Answer from the drawing. Dimensions are ordinates in mm from the lowest x, y and z of the part. Round coordinates to 2 decimals unless told otherwise and drop trailing zeros. Order: outer loops, then holes, each group sorted by start corner. A loop starts at its lowest first (then second) coordinate and runs counter-clockwise, first axis right, second up. Notation, with made-up numbers: (-3, 70) - (44, 70) arc R19 ccw to (44, 100) - close; hole circle Ø5 at (54.25, 61). An arc over 180 degrees is marked (long way). One line per question, with ' | ' between items. Start each with the question number.
1) The part is cut by section C-C, the plane x = 17. Give the vertices of the cut face in (y, z) (1 decimal).
2) Flat-ended cylindrical pins translate along their axes: pin 1 (5 mm diameter, centred on x = 22.5, z = 5, fed in from -Y); pin 2 (1.2 mm diameter, centred on x = 30, y = 1.5, fed in from -Z). Find the tip coordinate at first contact, or state that the pin passes through.
3) The mould has two halves that part along X. Classify the marked faces 1, 2 and 3: pulls with the +X half, pulls with the -X half, needs draft (parallel to the pull), parting line crosses it, or undercut.
4) The part is cut by section A-A, the plane x = 25. Give the vertices of the cut face in (y, z).
5) Straight lines are drawn through the part: line 1 (Z direction, x = 20, y = 1.75); line 2 (X direction, y = 1.1, z = 15.25) (1 decimal); line 3 (X direction, y = 2.3, z = 19.25) (1 decimal). For each, find the intervals that lie inside material, in ascending order. Write a range as from..to.
6) The part is cut by section B-B, the plane z = 14.75. Give the vertices of the cut face in (x, y) (1 decimal), plus the area to 3 significant figures.
7) The part is cut by section D-D, the plane y = 0.8. Count the separate pieces of the cut face and the enclosed holes in it.
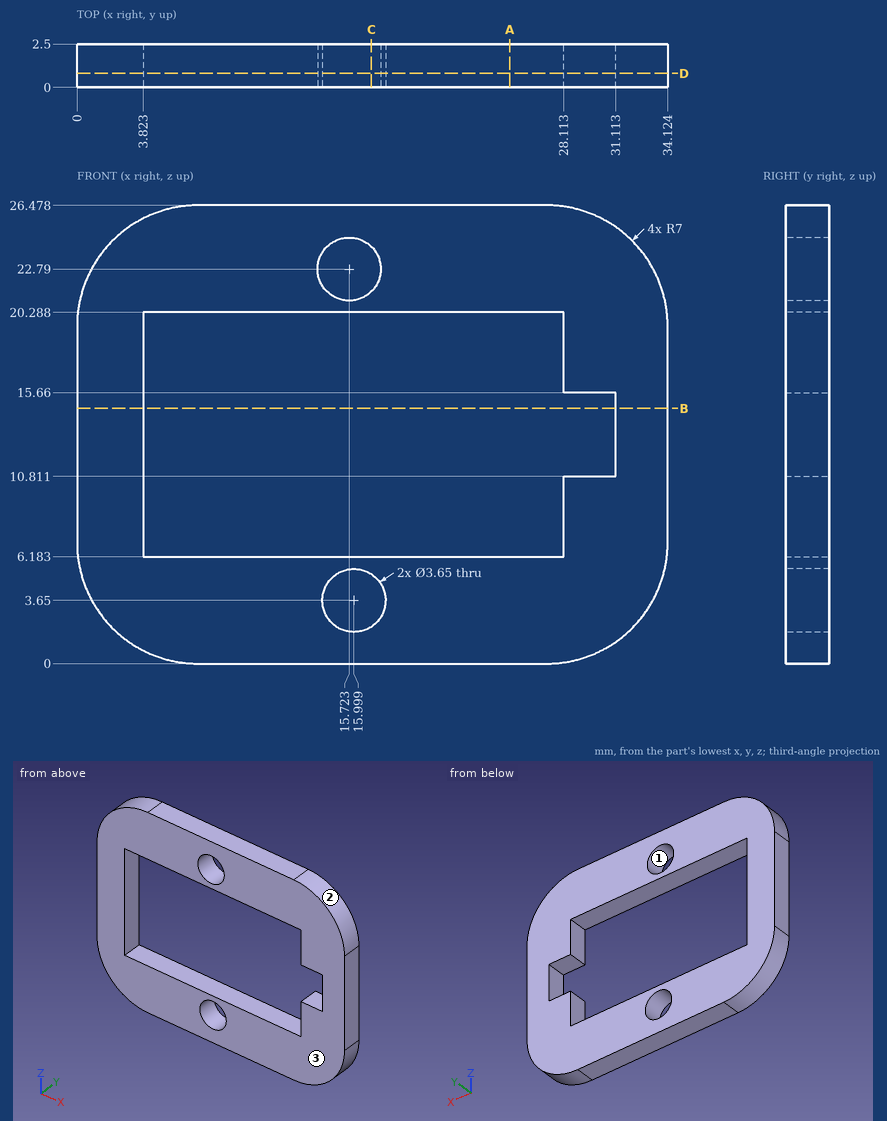
Values:
1) outline: (0, 0) - (2.5, 0) - (2.5, 2.1) - (0, 2.1) - close; (0, 5.2) - (2.5, 5.2) - (2.5, 6.2) - (0, 6.2) - close; (0, 20.3) - (2.5, 20.3) - (2.5, 21.5) - (0, 21.5) - close; (0, 24.1) - (2.5, 24.1) - (2.5, 26.5) - (0, 26.5) - close
2) pin 1: stops at y = 0 | pin 2: stops at z = 0.38
3) face 1: undercut | face 2: pulls with the +X half | face 3: needs draft
4) outline: (0, 0) - (2.5, 0) - (2.5, 6.18) - (0, 6.18) - close; (0, 20.29) - (2.5, 20.29) - (2.5, 26.48) - (0, 26.48) - close
5) line 1: z = 0..6.18, 20.29..26.48 | line 2: x = 0..3.8, 31.1..34.1 | line 3: x = 0..3.8, 28.1..34.1
6) outline: (0, 0) - (3.8, 0) - (3.8, 2.5) - (0, 2.5) - close; (31.1, 0) - (34.1, 0) - (34.1, 2.5) - (31.1, 2.5) - close | area: 17.1 mm^2
7) separate pieces: 1 | enclosed holes: 3
